Part model, mm, in its own coordinate system. A direction names the side the tool comes from. Round coordinates to 2 decimals unless told otherwise and drop trailing zeros.
Autodesk Inventor part; units mm, degrees
ref_plane "YZ Plane" through (0, 0, 0) normal (1, 0, 0) x (0, 1, 0)
ref_plane "XZ Plane" through (0, 0, 0) normal (0, 1, 0) x (-1, 0, 0)
ref_plane "XY Plane" through (0, 0, 0) normal (0, 0, 1) x (1, 0, 0)
sketch "Sketch1" plane through (0, 0, 0) normal (0, 0, 1) x (1, 0, 0)
  line L0 (0, 0) -> (-142, 0)
  line L1 (-142, 0) -> (-142, 218)
  line L2 (-142, 218) -> (0, 218)
  line L3 (0, 218) -> (0, 0)
  dimension "d0" = 142
  dimension "d1" = 218
extrude "Extrusion1" add sketch "Sketch1" along normal blind 67
sketch "Sketch6" plane through (-142, 218, 0) normal (0, 1, 0) x (1, 0, 0)
  line L0 (0, -67) -> (142, -67)
  line L1 (142, 0) -> (142, -67)
  line L2 (0, 0) -> (142, 0)
  line L3 (0, 0) -> (0, -67)
  line L4 (11, -9) -> (131, -9)
  line L5 (131, -9) -> (131, -58)
  line L6 (131, -58) -> (11, -58)
  line L7 (11, -58) -> (11, -9)
  dimension "d33" = 67
  dimension "d34" = 142
  dimension "d35" = 11
  dimension "d36" = 11
  dimension "d37" = 9
  dimension "d38" = 9
extrude "Extrusion5" cut sketch "Sketch6" against normal blind 4 contours L4 L5 L6 L7
sketch "Sketch7" plane through (-142, 214, 0) normal (0, 1, 0) x (1, 0, 0)
  line L0 (11, -58) -> (131, -58)
  line L1 (131, -58) -> (131, -9)
  line L2 (11, -9) -> (131, -9)
  line L3 (131, -9) -> (131, -58)
  line L4 (131, -58) -> (11, -58)
  line L5 (11, -58) -> (11, -9)
  line L6 (11, -9) -> (11, -32)
  line L7 (11, -32) -> (11, -35)
  line L8 (11, -35) -> (11, -58)
  line L9 (11, -32) -> (16, -32)
  line L10 (11, -35) -> (16, -35)
  line L11 (11, -9) -> (29, -9)
  line L12 (29, -9) -> (32, -9)
  line L13 (32, -9) -> (69.5, -9)
  line L14 (69.5, -9) -> (72.5, -9)
  line L15 (72.5, -9) -> (110, -9)
  line L16 (131, -9) -> (113, -9)
  line L17 (113, -9) -> (110, -9)
  line L18 (29, -9) -> (29, -18.5)
  line L19 (32, -18.5) -> (32, -9)
  line L20 (29, -9) -> (32, -9)
  line L21 (32, -58) -> (32, -48.5)
  line L22 (29, -48.5) -> (29, -58)
  line L23 (16, -48.5) -> (16, -35)
  line L24 (16, -32) -> (16, -18.5)
  line L25 (16, -18.5) -> (29, -18.5)
  line L26 (32, -18.5) -> (46, -18.5)
  line L27 (46, -18.5) -> (46, -32)
  line L28 (46, -35) -> (46, -48.5)
  line L29 (69.5, -9) -> (69.5, -32)
  line L30 (69.5, -35) -> (69.5, -58)
  line L31 (72.5, -9) -> (72.5, -32)
  line L32 (72.5, -35) -> (72.5, -58)
  line L33 (46, -32) -> (69.5, -32)
  line L34 (46, -35) -> (69.5, -35)
  line L35 (72.5, -35) -> (96, -35)
  line L36 (126, -35) -> (131, -35)
  line L37 (110, -9) -> (110, -18.5)
  line L38 (110, -48.5) -> (110, -58)
  line L39 (72.5, -32) -> (96, -32)
  line L40 (126, -32) -> (131, -32)
  line L41 (113, -9) -> (113, -18.5)
  line L42 (110, -58) -> (110, -48.5)
  line L43 (110, -18.5) -> (110, -9)
  line L44 (113, -48.5) -> (113, -58)
  line L45 (126, -48.5) -> (113, -48.5)
  line L46 (110, -48.5) -> (96, -48.5)
  line L47 (126, -18.5) -> (126, -32)
  line L48 (126, -35) -> (126, -48.5)
  line L49 (96, -48.5) -> (96, -35)
  line L50 (96, -32) -> (96, -18.5)
  line L51 (96, -18.5) -> (110, -18.5)
  line L52 (113, -18.5) -> (126, -18.5)
  line L53 (46, -48.5) -> (32, -48.5)
  line L54 (29, -48.5) -> (16, -48.5)
  line L55 (11, -32) -> (16, -32)
  line L56 (16, -18.5) -> (29, -18.5)
  line L57 (29, -9) -> (32, -9)
  line L58 (32, -18.5) -> (46, -18.5)
  line L59 (46, -32) -> (69.5, -32)
  line L60 (69.5, -9) -> (72.5, -9)
  line L61 (72.5, -32) -> (96, -32)
  line L62 (96, -18.5) -> (110, -18.5)
  line L63 (110, -9) -> (113, -9)
  line L64 (113, -18.5) -> (126, -18.5)
  line L65 (126, -32) -> (131, -32)
  line L66 (131, -35) -> (126, -35)
  line L67 (126, -48.5) -> (113, -48.5)
  line L68 (113, -58) -> (110, -58)
  line L69 (110, -48.5) -> (96, -48.5)
  line L70 (96, -35) -> (72.5, -35)
  line L71 (72.5, -58) -> (69.5, -58)
  line L72 (69.5, -35) -> (46, -35)
  line L73 (46, -48.5) -> (32, -48.5)
  line L74 (32, -58) -> (29, -58)
  line L75 (29, -48.5) -> (16, -48.5)
  line L76 (16, -35) -> (11, -35)
  point P0 (142, 0)
extrude "Extrusion6" add sketch "Sketch7" along normal blind 1 contours L22 L54 L23 L10 L5 L9 L24 L25 L18 L2 L19 L26 L27 L33 L29 L31 L39 L50 L51 L37 L41 L52 L47 L40 L1 L36 L48 L45 L44 L0 L38 L46 L49 L35 L32 L30 L34 L28 L53 L21
sketch "Sketch8" plane through (-142, 215, 0) normal (0, 1, 0) x (1, 0, 0)
  line L0 (126, -18.5) -> (126, -32)
  line L1 (113, -18.5) -> (126, -18.5)
  line L2 (32, -18.5) -> (46, -18.5)
  line L3 (16, -32) -> (16, -18.5)
  line L4 (31, -47.3564) -> (19, -40.4282)
  line L5 (19, -40.4282) -> (19, -26.5718)
  line L6 (19, -26.5718) -> (31, -19.6436)
  line L7 (31, -19.6436) -> (43, -26.5718)
  line L8 (43, -26.5718) -> (43, -40.4282)
  line L9 (43, -40.4282) -> (31, -47.3564)
  line L10 (110.8321, -19.6446) -> (122.9152, -26.4269)
  line L11 (122.9152, -26.4269) -> (123.0831, -40.2823)
  line L12 (123.0831, -40.2823) -> (111.1679, -47.3554)
  line L13 (111.1679, -47.3554) -> (99.0848, -40.5731)
  line L14 (99.0848, -40.5731) -> (98.9169, -26.7177)
  line L15 (98.9169, -26.7177) -> (110.8321, -19.6446)
  circle A0 centre (111, -33.5) radius 3.75
  circle A1 centre (31, -33.5) radius 3.75
  circle A2 centre (71, -33.5) radius 14
  point P0 (142, 0)
  dimension "d62" = 15
  dimension "d63" = 15
  dimension "d64" = 15
  dimension "d65" = 15
  dimension "d66" = 12
  dimension "d67" = 12
  dimension "d69" = 7.5
  dimension "d70" = 7.5
  dimension "d71" = 28
extrude "Extrusion7" add sketch "Sketch8" along normal blind 4 contours L4 L5 L6 L7 L8 L9 | L10 L11 L12 L13 L14 L15 | A0 | A1 | A2
sketch "Sketch9" plane through (-71, 219, 33.5) normal (0, 1, 0) x (1, 0, 0)
  circle A0 centre (0, 0) radius 14
  circle A1 centre (0, 0) radius 12.5
  point P0 (71, 33.5)
  dimension "d74" = 25
extrude "Extrusion8" cut sketch "Sketch9" against normal blind 0.5 contours A1
sketch "Sketch10" plane through (-71, 218.5, 33.5) normal (0, 1, 0) x (1, 0, 0)
  circle A0 centre (0, 0) radius 12.5
  line L0 (0, 4.6188) -> (4, 2.3094)
  line L1 (4, 2.3094) -> (4, -2.3094)
  line L2 (4, -2.3094) -> (0, -4.6188)
  line L3 (0, -4.6188) -> (-4, -2.3094)
  line L4 (-4, -2.3094) -> (-4, 2.3094)
  line L5 (-4, 2.3094) -> (0, 4.6188)
  circle A1 centre (0, 0) radius 1.5
  point P0 (71, 33.5)
  dimension "d77" = 4
  dimension "d78" = 3
extrude "Extrusion9" cut sketch "Sketch10" against normal blind 1 contours L0 L1 L2 L3 L4 L5 | A1
sketch "Sketch11" plane through (-71, 217.5, 33.5) normal (0, 1, 0) x (1, 0, 0)
  circle A0 centre (0, 0) radius 1.5
  point P0 (71, 33.5)
  dimension "d81" = 3
extrude "Extrusion10" cut sketch "Sketch11" against normal blind 0.1
sketch "Sketch13" plane through (-142, 219, 0) normal (0, 1, 0) x (1, 0, 0)
  circle A0 centre (31, -33.5) radius 2.5
  point P0 (142, 0)
  dimension "d84" = 5
extrude "Extrusion11" cut sketch "Sketch13" against normal blind 8
sketch "Sketch14" plane through (-142, 219, 0) normal (0, 1, 0) x (1, 0, 0)
  circle A0 centre (111, -33.5) radius 2.5
  point P0 (142, 0)
  dimension "d87" = 5
extrude "Extrusion12" cut sketch "Sketch14" against normal blind 8
equation "\"BendRadius\" = Thickness"
equation "\"BendReliefWidth\" = Thickness"
equation "\"BendReliefDepth\" = 0.5 * Thickness"
equation "\"CornerReliefSize\" = 4 * Thickness"
equation "\"MinimumRemnant\" = 2 * Thickness"
equation "\"TransitionRadius\" = BendRadius"
equation "\"JacobiRadiusSize\" = Thickness"
equation "\"GapSize\" = Thickness"
properties part number "CALB100AH final"
1) Drop flat-ended pins along their axis: pin 1 Ø5 at (x, z) = (-45.5, 14.5) entering from +Y; pin 2 Ø2.5 at (x, z) = (-72.5, 32) entering from +Y. Give the stop position or say it passes through.
Values:
pin 1: stops at y = 214
pin 2: stops at y = 217.5
2) Tool access for faces 1 (the face through (-70, 0, 33)), 2 (the face through (-55, 214, 46)), 3 (the face through (-104.916, 216.972, 43.844)): list every direction of +Z, -Z, +X, -X, +Y, -Y with a clear straight run to the whole face (end or side of a thin tool).
Values:
face 1: +Z, -Z, +X, -X, -Y
face 2: none
face 3: +Y
3) Mould opens along Z. For faces 4 (the face through (-18, 214, 51)), 5 (the face through (-111.2, 219, 36.4)), 6 (the face through (-72, 111, 67)) say: released by +Z, released by -Z, zero draft, split by the parting line, or undercut.
Values:
face 4: undercut
face 5: zero draft
face 6: released by +Z
4) Wall check: line 1 along X through (y, z) = (213, 33.5); line 2 along X through (y, z) = (213, 33); line 3 along Z through (x, y) = (-71, 217.45). Give the ranges that are in metal, low to high.
Values:
line 1: x = -142 to -113.5, -108.5 to -33.5, -28.5 to 0
line 2: x = -142 to -113.45, -108.55 to -33.45, -28.55 to 0
line 3: z = 0 to 9, 19.5 to 32, 35 to 47.5, 58 to 67
